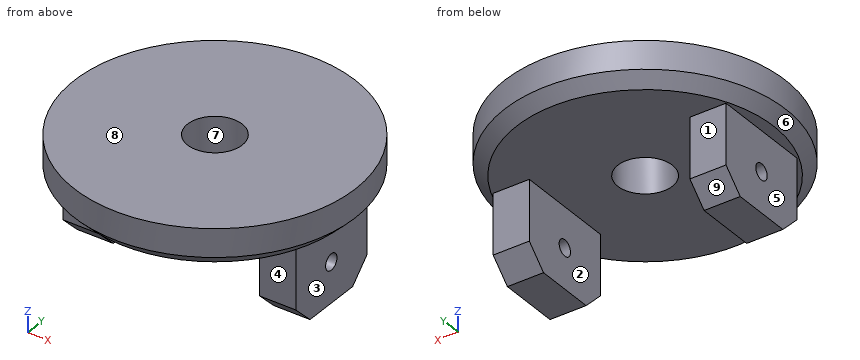
```python
from build123d import *

# Parameters (mm, degrees)
F1_DEPTH  = 5
F3_SIZE   = 1
F2_W      = 4.5
F2_H      = 12.5
F4_DEPTH  = 10
F5_SIZE   = 2.5
F6_R      = 1
F7_DEPTH  = 39.5010001
F8_R      = 39.5864097355
F8_R_2    = 17.5
F9_DEPTH  = 25
F10_SIZE  = 1.5
F11_R     = 3.4
F12_DEPTH = 25


with BuildPart() as f1:
    # F0 (on Top) → F1 (new body)
    with BuildSketch(Plane.XY):
        with BuildLine():
            ThreePointArc((19.8625961196, -15.8301909188), (23.6080012184, -12.5093598908), (25, -7.7012087429))
            Line((25, -7.7012087429), (25, 7.7012087429))
            ThreePointArc((25, 7.7012087429), (23.6080012184, 12.5093598908), (19.8625961196, 15.8301909188))
            add(Edge.make_bspline(
                [(19.8625961196, 15.8301909188), (0, 25.2681728257), (-19.8625961196, 15.8301909188)],
                knots=[0.9132750433, 0.9132750433, 0.9132750433, 2.2283176103, 2.2283176103, 2.2283176103], degree=2, weights=[1, 0.7915095459, 1]))
            ThreePointArc((-19.8625961196, 15.8301909188), (-23.6080012184, 12.5093598908), (-25, 7.7012087429))
            Line((-25, 7.7012087429), (-25, -7.7012087429))
            ThreePointArc((-25, -7.7012087429), (-23.6080012184, -12.5093598908), (-19.8625961196, -15.8301909188))
            add(Edge.make_bspline(
                [(-19.8625961196, -15.8301909188), (0, -25.2681728257), (19.8625961196, -15.8301909188)],
                knots=[4.0548676969, 4.0548676969, 4.0548676969, 5.3699102639, 5.3699102639, 5.3699102639], degree=2, weights=[1, 0.7915095459, 1]))
        make_face()
    extrude(amount=F1_DEPTH)

    # F3
    f3_edges = [f1.edges().sort_by_distance(p)[0] for p in [
        (4e-06, -20, 0),
    ]]
    chamfer(f3_edges, length=F3_SIZE)

    # F2 (on face) → F4 (join)
    with BuildSketch(Plane(origin=(0, 0, 0), x_dir=(1, 0, 0), z_dir=(0, 0, -1))):
        with Locations((12.25, 0)):
            Rectangle(F2_W, F2_H)
        with Locations((-12.25, 0)):
            Rectangle(F2_W, F2_H)
    extrude(amount=F4_DEPTH)

    # F5
    f5_edges = [f1.edges().sort_by_distance(p)[0] for p in [
        (-12.25, -6.25, -10),
        (12.25, -6.25, -10),
        (-12.25, 6.25, -10),
        (12.25, 6.25, -10),
    ]]
    chamfer(f5_edges, length=F5_SIZE)

    # F6 (on face) → F7 (cut, through all)
    with BuildSketch(Plane.YZ.offset(14.5)):
        with Locations((0, -5)):
            Circle(F6_R)
    extrude(amount=-F7_DEPTH, mode=Mode.SUBTRACT)

    # F8 (on face) → F9 (cut)
    with BuildSketch(Plane.XY.offset(5)):
        Circle(F8_R)
        with BuildLine():
            add(Edge.make_bspline(
                [(-19.8625961196, -15.8301909188), (0, -25.2681728257), (19.8625961196, -15.8301909188)],
                knots=[4.0548676969, 4.0548676969, 4.0548676969, 5.3699102639, 5.3699102639, 5.3699102639], degree=2, weights=[1, 0.7915095459, 1]))
            ThreePointArc((-19.8625961196, -15.8301909188), (-23.6080012184, -12.5093598908), (-25, -7.7012087429))
            Line((-25, -7.7012087429), (-25, 7.7012087429))
            ThreePointArc((-25, 7.7012087429), (-23.6080012184, 12.5093598908), (-19.8625961196, 15.8301909188))
            add(Edge.make_bspline(
                [(19.8625961196, 15.8301909188), (0, 25.2681728257), (-19.8625961196, 15.8301909188)],
                knots=[0.9132750433, 0.9132750433, 0.9132750433, 2.2283176103, 2.2283176103, 2.2283176103], degree=2, weights=[1, 0.7915095459, 1]))
            ThreePointArc((19.8625961196, 15.8301909188), (23.6080012184, 12.5093598908), (25, 7.7012087429))
            Line((25, 7.7012087429), (25, -7.7012087429))
            ThreePointArc((25, -7.7012087429), (23.6080012184, -12.5093598908), (19.8625961196, -15.8301909188))
        make_face(mode=Mode.SUBTRACT)
        with BuildLine():
            ThreePointArc((-25, -7.7012087429), (-23.6080012184, -12.5093598908), (-19.8625961196, -15.8301909188))
            add(Edge.make_bspline(
                [(-19.8625961196, -15.8301909188), (0, -25.2681728257), (19.8625961196, -15.8301909188)],
                knots=[4.0548676969, 4.0548676969, 4.0548676969, 5.3699102639, 5.3699102639, 5.3699102639], degree=2, weights=[1, 0.7915095459, 1]))
            ThreePointArc((19.8625961196, -15.8301909188), (23.6080012184, -12.5093598908), (25, -7.7012087429))
            Line((25, -7.7012087429), (25, 7.7012087429))
            ThreePointArc((25, 7.7012087429), (23.6080012184, 12.5093598908), (19.8625961196, 15.8301909188))
            add(Edge.make_bspline(
                [(19.8625961196, 15.8301909188), (0, 25.2681728257), (-19.8625961196, 15.8301909188)],
                knots=[0.9132750433, 0.9132750433, 0.9132750433, 2.2283176103, 2.2283176103, 2.2283176103], degree=2, weights=[1, 0.7915095459, 1]))
            ThreePointArc((-19.8625961196, 15.8301909188), (-23.6080012184, 12.5093598908), (-25, 7.7012087429))
            Line((-25, 7.7012087429), (-25, -7.7012087429))
        make_face()
        Circle(F8_R_2, mode=Mode.SUBTRACT)
    extrude(amount=-F9_DEPTH, mode=Mode.SUBTRACT)

    # F10
    f10_edges = [f1.edges().sort_by_distance(p)[0] for p in [
        (-17.5, 0, 0),
    ]]
    chamfer(f10_edges, length=F10_SIZE)

    # F11 (on face) → F12 (cut)
    with BuildSketch(Plane.XY.offset(5)):
        Circle(F11_R)
    extrude(amount=-F12_DEPTH, mode=Mode.SUBTRACT)


solid = f1.part
```
The listing builds one solid part. Answer for the finished solid, in the listing's coordinates (mm). Face numbers are marked on the shaded views. A direction names the side the tool comes from. Coordinates: 2 decimals unless noted, no trailing zeros. Loops run counter-clockwise (first coordinate to the right, second up) from the corner with the lowest first, then second, coordinate; pieces in that order, holes last. Notation, with made-up numbers: (16.5, 87.25) -> (56.5, 87.25) arc R14 ccw to (56.5, 95.25) -> close; hole circle Ø8 at (-29, 45). An arc over 180 degrees is marked (long way). Return JSON: item names as keys, results as strings. Group by question number.
(1) A cutting plane is placed at B-B on x = 0. Write down the section's boundary in (y, z), and give its area (3 significant figures).
(2) A cutting plane is placed at A-A on y = 0. Write down the section's boundary in (x, z).
(3) Determine the mould class of the marked faces 6, 7, 8 and 9 for opening direction Y: released by +Y, released by -Y, zero draft, split by the parting line, or undercut.
(4) Which of the six approach directions +Z, -Z, +X, -X, +Y, -Y give full straight-line access (tool end or side, diameter ignored) to the marked faces 1, 2, 3, 4 and 5?
(5) A cutting plane is placed at C-C on z = -5. Write down the section's boundary in (x, y), and give its area (3 significant figures).
(6) Find the intervals of material crossed by probe 1 along Y at (x, z) = (0, 3.5); probe 2 along X at (y, z) = (-6, -6.5); probe 3 along Z at (x, y) = (9, -9), in increasing order. Write a range as from..to.
(7) Given pin 1 Ø3 at (y, z) = (0, -5) entering from -X; pin 2 Ø5 at (x, z) = (-13, -3) entering from +Y; pin 3 Ø4 at (x, y) = (0, 0) entering from +Z (3 decimals); pin 4 Ø3 at (y, z) = (-1, -5) entering from +X, each flat-ended and moving along its own axis, determine where each tip first touches the part or whether it passes through.
The answers:
{
 "1": {"outline": "(-17.5, 1.5) -> (-16, 0) -> (-3.4, 0) -> (-3.4, 5) -> (-17.5, 5) -> close; (3.4, 0) -> (16, 0) -> (17.5, 1.5) -> (17.5, 5) -> (3.4, 5) -> close", "area": "139 mm^2"},
 "2": {"outline": "(-17.5, 1.5) -> (-16, 0) -> (-14.5, 0) -> (-14.5, -4) -> (-10, -4) -> (-10, 0) -> (-3.4, 0) -> (-3.4, 5) -> (-17.5, 5) -> close; (-14.5, -10) -> (-10, -10) -> (-10, -6) -> (-14.5, -6) -> close; (3.4, 0) -> (10, 0) -> (10, -4) -> (14.5, -4) -> (14.5, 0) -> (16, 0) -> (17.5, 1.5) -> (17.5, 5) -> (3.4, 5) -> close; (10, -10) -> (14.5, -10) -> (14.5, -6) -> (10, -6) -> close"},
 "3": {"face 6": "split by the parting line", "face 7": "undercut", "face 8": "zero draft", "face 9": "released by +Y"},
 "4": {"face 1": "-Z, +X, -X, +Y", "face 2": "-Z, +Y, -Y", "face 3": "-Z, +X, +Y, -Y", "face 4": "-Z, +X, -X, -Y", "face 5": "-Z, -X, +Y, -Y"},
 "5": {"outline": "(-14.5, -6.25) -> (-10, -6.25) -> (-10, -1) -> (-14.5, -1) -> close; (-14.5, 1) -> (-10, 1) -> (-10, 6.25) -> (-14.5, 6.25) -> close; (10, -6.25) -> (14.5, -6.25) -> (14.5, -1) -> (10, -1) -> close; (10, 1) -> (14.5, 1) -> (14.5, 6.25) -> (10, 6.25) -> close", "area": "94.5 mm^2"},
 "6": {"probe 1": "y = -17.5..-3.4, 3.4..17.5", "probe 2": "x = -14.5..-10, 10..14.5", "probe 3": "z = 0..5"},
 "7": {"pin 1": "stops at x = -14.5", "pin 2": "stops at y = 6.25", "pin 3": "passes through", "pin 4": "stops at x = 14.5"}
}
